Here's how the part is built. I have some questions about the finished solid (model axes, mm). A direction names the side the tool comes from. Round coordinates to 2 decimals unless told otherwise and drop trailing zeros. Loops run counter-clockwise (first coordinate to the right, second up) from the corner with the lowest first, then second, coordinate; pieces in that order, holes last. Notation, with made-up numbers: M 35.25,66 L 71.25,66 A25 cw 71.25,89 Z; hole C 65.25,6 d6. An arc over 180 degrees is marked long. Answer as a JSON object with one key per item and string values.
from build123d import *

# Parameters (mm, degrees)
BASPROSKE_W      = 3
BASPROSKE_H      = 5.5
TOOTHCUT_DEPTH   = 9.336666
TEETHCUTS_COUNT  = 20
TEETHCUTS_ANGLE  = 342
HUBNEAONESKE_R   = 4
HUBNEARONE_DEPTH = 5.0000508
BORSKE_R         = 2
BORE_DEPTH       = 8.0000508


with BuildPart() as part:
    # BasProSke → Base-Revolve (revolve)
    with BuildSketch(Plane(origin=(0, 0, 0), x_dir=(1, 0, 0), z_dir=(0, 1, 0)), mode=Mode.PRIVATE) as base_revolve_sk:
        with Locations((1.5, 2.75)):
            Rectangle(BASPROSKE_W, BASPROSKE_H)
    revolve(base_revolve_sk.sketch.rotate(Axis((-10, 0, 0), (1, 0, 0)), 180), axis=Axis((-10, 0, 0), (1, 0, 0)))

    # TooCutSke → ToothCut (cut, through all)
    with BuildSketch(Plane(origin=(0, 0, 0), x_dir=(0, 0, -1), z_dir=(1, 0, 0))):
        with BuildLine():
            ThreePointArc((0.249903181, 4.366855207), (0, 4.374), (-0.249903181, 4.366855207))
            ThreePointArc((-0.249903181, 4.366855207), (-0.415207844, 4.95951031), (-0.752843848, 5.473871692))
            ThreePointArc((-0.752843848, 5.473871692), (0, 5.5254), (0.752843848, 5.473871692))
            ThreePointArc((0.752843848, 5.473871692), (0.415207844, 4.95951031), (0.249903181, 4.366855207))
        make_face()
    toothcut = extrude(amount=TOOTHCUT_DEPTH, mode=Mode.SUBTRACT)

    # TeethCuts: ToothCut ×20 about axis
    teethcuts_axis = Axis((-10, 0, 0), (1, 0, 0))
    for i in range(1, TEETHCUTS_COUNT):
        add(toothcut.rotate(teethcuts_axis, i * TEETHCUTS_ANGLE / (TEETHCUTS_COUNT - 1)), mode=Mode.SUBTRACT)

    # HubNeaOneSke → HubNearOne (add)
    with BuildSketch(Plane.ZY):
        with Locations(Location((0, 0, 0), (0, 0, 180))):
            Circle(HUBNEAONESKE_R)
    extrude(amount=HUBNEARONE_DEPTH)

    # BorSke → Bore (cut, symmetric)
    with BuildSketch(Plane(origin=(0, 0, 0), x_dir=(0, 0, -1), z_dir=(1, 0, 0))):
        with Locations(Location((0, 0, 0), (0, 0, 180))):
            Circle(BORSKE_R)
    extrude(amount=BORE_DEPTH, both=True, mode=Mode.SUBTRACT)


solid = part.part
Item 1: I want a section at C-C, the plane z = 3. Please give me the cut outline in (x, y), then the cut area to 3 significant figures.
Resolved:
{"outline": "M -5,-2.65 L 0,-2.65 L 0,-3.6 L 3,-3.6 L 3,3.6 L 0,3.6 L 0,2.65 L -5,2.65 Z", "area": "48.1 mm²"}
Item 2: I'm going to push flat-ended pins straight in: pin 1 Ø1.5 at (x, y) = (-3.5, 3) entering from -Z; pin 2 Ø1.5 at (x, z) = (-3.5, -2.5) entering from -Y; pin 3 Ø4 at (x, z) = (-4, 0) entering from -Y. Where does each tip first touch, or does it pass through?
Resolved:
{"pin 1": "z = -3.31", "pin 2": "y = -3.6", "pin 3": "y = -4"}
Item 3: Please list where these lines run through material, in increasing order: probe 1 along Y at (x, z) = (-1.75, 0); probe 2 along Z at (x, y) = (2.25, 3.5); probe 3 along X at (y, z) = (5, -0.5). Write a range as from..to.
Resolved:
{"probe 1": "-4..-2, 2..4", "probe 2": "-3.89..-2.88, -2.62..2.62, 2.88..3.89", "probe 3": "0..3"}
Item 4: I want a section at A-A, the plane z = 0. Please give me the cut outline in (x, y), then the cut area to 3 significant figures.
Resolved:
{"outline": "M -5,-4 L 0,-4 L 0,-4.37 L 3,-4.37 L 3,-2 L -5,-2 Z; M -5,2 L 3,2 L 3,4.37 L 0,4.37 L 0,4 L -5,4 Z", "area": "34.2 mm²"}
Item 5: If we mould it in two halves opening along Y, with no side actions, what happens to faces 1 (the face through (1.479, -2.578, 4.25)), 2 (the face through (1.48, 4.57, 1.91)), 3 (the face through (1.479, -3.765, 3.245))? For each: pulls with the +Y half, pulls with the -Y half, needs draft (parallel to the pull), parting line crosses it, or undercut.
Resolved:
{"face 1": "undercut", "face 2": "pulls with the +Y half", "face 3": "pulls with the -Y half"}
Item 6: On a 3-axis mill with a long thin cutter (end or side, diameter ignored), from which of +Z, -Z, +X, -X, +Y, -Y can I reach the whole of each face in a straight line? I mean faces 4 (the face through (1.479, 3.756, 3.23)), 5 (the face through (1.48, 1.91, -4.57)), 6 (the face through (1.479, 2.578, -4.25)), 7 (the face through (1.479, -3.756, -3.23)). Say none if no direction works.
Resolved:
{"face 4": "+X, -X, +Y", "face 5": "-Z, +X, -X", "face 6": "+X, -X", "face 7": "+X, -X, -Y"}
